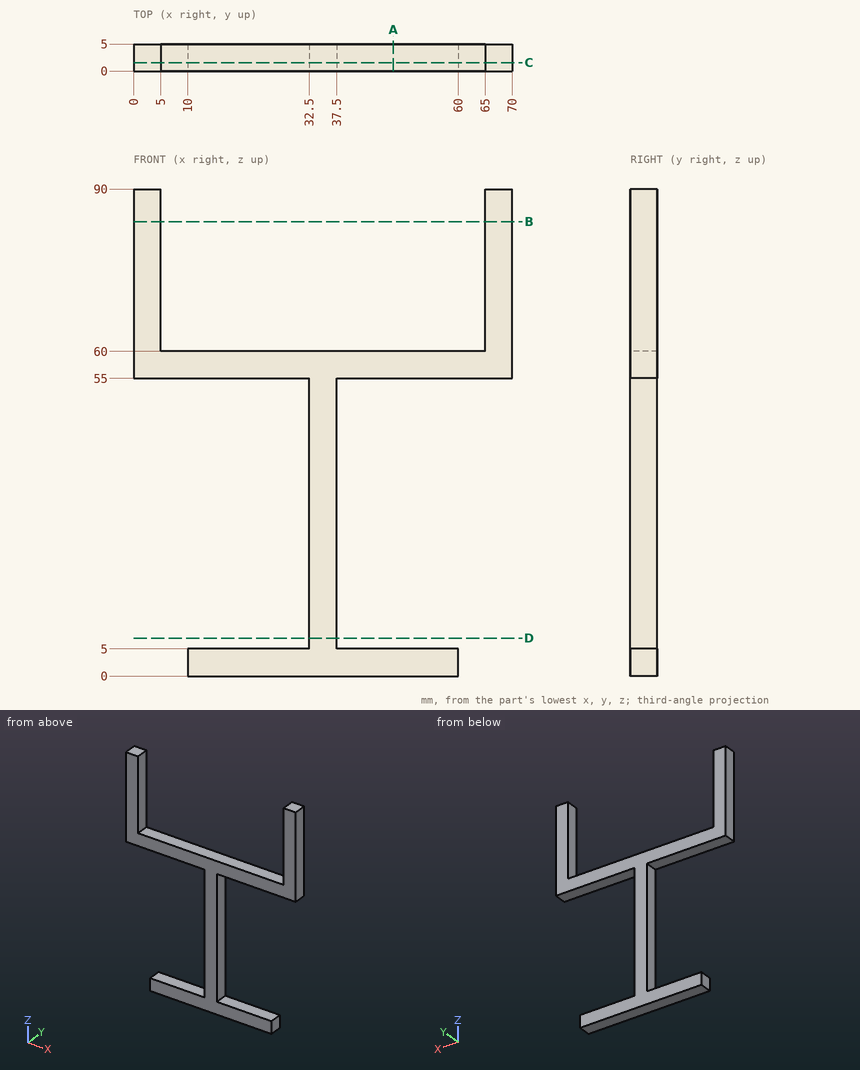
Could you check a few things on this drawing? It's one solid part, dimensions in mm from its lowest x, y, z. Give positions to 0.01 mm unless a question says otherwise; leave off trailing zeros. Order: outer loops, then holes, each group sorted by start corner. A loop starts at its lowest first (then second) coordinate and runs counter-clockwise, first axis right, second up. Notation, with made-up numbers: (66, 13) -> (112, 13) arc R22 cw to (112, 26) -> close; hole circle Ø2 at (50, 7). An arc over 180 degrees is marked (long way). Use CSV: the item, a comma, the result in double quotes. Start each with the question number.
Item 1: Suppose I cut it at A-A (x = 48). List the corners of the cut face in (y, z) for me, and give its area (3 significant figures).
Item 2: If I drill on probe 1 along Z at (x, y) = (52, 3.4); probe 2 along X at (y, z) = (3.6, 75.5); probe 3 along X at (y, z) = (0.95, 9.5), over which ranges is the centre line in solid material (lowest first)? Write a range as [from, to].
Item 3: Suppose I cut it at C-C (y = 1.55). List the corners of the cut face in (x, z) for me, and give its area (3 significant figures).
Item 4: I'm going to push flat-ended pins straight in: P1, Ø1.5, axis at y = 3.5, z = 50, coming from the -X side; P2, Ø1.5, axis at x = 53.5, y = 1.5, coming from the +Z side; P3, Ø2.5, axis at y = 2, z = 2, coming from the -X side. Where does each tip first touch, or does it pass through?
Item 5: Suppose I cut it at D-D (z = 7). List the corners of the cut face in (x, y) for me.
Item 6: Suppose I cut it at B-B (z = 84). List the corners of the cut face in (x, y) for me, and give its area (3 significant figures).
Answer block:
1,outline,"(0, 0) -> (5, 0) -> (5, 5) -> (0, 5) -> close; (0, 55) -> (5, 55) -> (5, 60) -> (0, 60) -> close"
1,area,"50.0 mm^2"
2,probe 1,"z = [0, 5], [55, 60]"
2,probe 2,"x = [0, 5], [65, 70]"
2,probe 3,"x = [32.5, 37.5]"
3,outline,"(0, 55) -> (32.5, 55) -> (32.5, 5) -> (10, 5) -> (10, 0) -> (60, 0) -> (60, 5) -> (37.5, 5) -> (37.5, 55) -> (70, 55) -> (70, 90) -> (65, 90) -> (65, 60) -> (5, 60) -> (5, 90) -> (0, 90) -> close"
3,area,"1,150 mm^2"
4,P1,"stops at x = 32.5"
4,P2,"stops at z = 60"
4,P3,"stops at x = 10"
5,outline,"(32.5, 0) -> (37.5, 0) -> (37.5, 5) -> (32.5, 5) -> close"
6,outline,"(0, 0) -> (5, 0) -> (5, 5) -> (0, 5) -> close; (65, 0) -> (70, 0) -> (70, 5) -> (65, 5) -> close"
6,area,"50.0 mm^2"
